The listing builds one solid part. Answer for the finished solid, in the listing's coordinates (mm). A direction names the side the tool comes from. Coordinates: 2 decimals unless noted, no trailing zeros. Order: outer loops, then holes, each group sorted by start corner. A loop starts at its lowest first (then second) coordinate and runs counter-clockwise, first axis right, second up. Notation, with made-up numbers: (78, -7.5) -> (134, -7.5) arc R10 cw to (134, 8.5) -> close; hole circle Ø11 at (3.5, 87). An arc over 180 degrees is marked (long way). Return JSON: item names as keys, results as strings.
Autodesk Inventor part; units mm, degrees
ref_plane "YZ Plane" through (0, 0, 0) normal (1, 0, 0) x (0, 1, 0)
ref_plane "XZ Plane" through (0, 0, 0) normal (0, 1, 0) x (-1, 0, 0)
ref_plane "XY Plane" through (0, 0, 0) normal (0, 0, 1) x (1, 0, 0)
sketch "スケッチ1" plane through (0, 0, 0) normal (0, 1, 0) x (-1, 0, 0)
  circle A0 centre (0, 0) radius 9
  line L0 (18, 10) -> (-18, 10)
  line L1 (-18, 10) -> (-18, -18)
  line L2 (-18, -18) -> (18, -18)
  line L3 (18, -18) -> (18, 10)
  line L4 (18, 30) -> (-18, 30)
  line L5 (-18, 30) -> (-18, 10)
  line L6 (-18, 10) -> (18, 10)
  line L7 (18, 10) -> (18, 30)
  line L8 (18, 30) -> (-18, 10) construction
  line L9 (-18, 30) -> (18, 10) construction
  point P0 (0, 20)
  point P1 (0, 20)
  point P2 (20, 10)
  point P3 (-6.6332, 10)
  point P4 (6.6332, 10)
  dimension "d0" = 18
  dimension "d18" = 10
  dimension "d33" = 30
  dimension "d34" = 36
  dimension "d36" = 18
extrude "押し出し1" add sketch "スケッチ1" along normal mid plane 10
sketch "スケッチ2" plane through (-38, 5, 30) normal (0, 0, 1) x (1, 0, 0)
  line L0 (20, -10) -> (20, 0)
  line L1 (56, -10) -> (20, -10)
  line L2 (56, 0) -> (56, -10)
  point P0 (38, -5)
  point P1 (25, -5)
  point P2 (51, -5)
  dimension "d37" = 5
  dimension "d38" = 5
  dimension "d39" = 5
hole "穴1" at (-13, 0, 30) at (13, 0, 30) direction (0, 0, -1) diameter 5 depth 6 tip angle 118
fillet "フィレット1" radius 10 2 edges at (18, 0, -18) (-18, 0, -18)
sketch "スケッチ4" plane through (0, 5, 0) normal (0, 1, 0) x (1, 0, 0)
  circle A0 centre (0, 0) radius 13
  circle A1 centre (0, 0) radius 9
  dimension "d43" = 26
extrude "押し出し3" add sketch "スケッチ4" along normal blind 16
chamfer "面取り3" distance 0.5 angle 45 2 edges at (-9, 21, 0) (-13, 21, 0)
properties part number "cable_holder" material "ABS プラスチック"
1. The part is cut by section B-B on x = 0. Give the vertices of the cut face in (y, z), and give its area (4 significant figures).
Answer block:
{"outline": "(-5, -18) -> (5, -18) -> (5, -13) -> (20.5, -13) -> (21, -12.5) -> (21, -9.5) -> (20.5, -9) -> (-5, -9) -> close; (-5, 9) -> (20.5, 9) -> (21, 9.5) -> (21, 12.5) -> (20.5, 13) -> (5, 13) -> (5, 30) -> (-5, 30) -> close", "area": "427.5 mm2"}
2. The part is cut by section C-C on y = 6.5. Give the vertices of the cut face in (x, z), and give its area (3 significant figures).
Answer block:
{"outline": "circle Ø26 at (0, 0); hole circle Ø18 at (0, 0)", "area": "276 mm2"}
3. Determine the mould class of faces 4 (the face through (0, -5, 12)), 5 (the face through (-10.316, 12.642, -7.91)), 6 (the face through (13.37, -0.23, 22.76)) for opening direction Y: pulls with the +Y half, pulls with the -Y half, needs draft (parallel to the pull), parting line crosses it, or undercut.
Answer block:
{"face 4": "pulls with the -Y half", "face 5": "needs draft", "face 6": "undercut"}
4. The part is cut by section A-A on z = 0. Give the vertices of the cut face in (x, y).
Answer block:
{"outline": "(-18, -5) -> (-9, -5) -> (-9, 20.5) -> (-9.5, 21) -> (-12.5, 21) -> (-13, 20.5) -> (-13, 5) -> (-18, 5) -> close; (9, -5) -> (18, -5) -> (18, 5) -> (13, 5) -> (13, 20.5) -> (12.5, 21) -> (9.5, 21) -> (9, 20.5) -> close"}
5. Each of these flat-tipped pins is pushed along its axis until it touches: pin 1 Ø8 at (x, z) = (2, 18) entering from +Y; pin 2 Ø4 at (x, y) = (-9, 10.5) entering from -Z; pin 3 Ø8 at (x, y) = (-13, 0) entering from -Z; pin 4 Ø16 at (x, z) = (0, 0) entering from -Y. Where does it stop, or does it pass through?
Answer block:
{"pin 1": "stops at y = 5", "pin 2": "stops at z = -10.95", "pin 3": "stops at z = -17.95", "pin 4": "passes through"}
6. Consider line 1 (X direction, y = 0, z = 28.15); line 2 (Z direction, x = 0, y = -1.25); line 3 (Y direction, x = 13, z = 26). Determine where each line is inside the solid, lowest interval first. Write a range as from..to.
Answer block:
{"line 1": "x = -18..-15.5, -10.5..10.5, 15.5..18", "line 2": "z = -18..-9, 9..30", "line 3": "y = -5..-2.5, 2.5..5"}
7. For faces 1 (the face through (15.44, 0.54, 26.96)), 2 (the face through (0, 0, 30)), 3 (the face through (0, 5, 17)), determine the directions among +Z, -Z, +X, -X, +Y, -Y from which every point of the face is accessible in a straight line to the end or side of a thin tool.
Answer block:
{"face 1": "+Z", "face 2": "+Z, +X, -X, +Y, -Y", "face 3": "+Y"}
